Answer from the drawing. Dimensions are ordinates in mm from the lowest x, y and z of the part. Coordinates: 2 decimals unless noted, no trailing zeros. Write each loop counter-clockwise with the first axis right and the second up, starting at its lowest first coordinate (ties: lowest second). Pieces come first, ordered by that corner, then holes.
(1) Given pin 1 (5 mm diameter, centred on y = 18, z = 8.5, fed in from +X); pin 2 (4 mm diameter, centred on x = 69, z = 6, fed in from -Y); pin 3 (1.5 mm diameter, centred on y = 25, z = 3.5, fed in from +X) (1 decimal); pin 4 (4 mm diameter, centred on x = 96.5, z = 9.5, fed in from +Y), each flat-ended and moving along its own axis, determine where each tip first touches the part or whether it passes through.
(2) The part is cut by section D-D, the plane z = 2. Determine the outline of the cut face in (x, y) (1 decimal), and give its area (3 significant figures).
(3) Determine the mould class of the marked faces 1, 2, 3 and 4 for opening direction X: pulls with the +X half, pulls with the -X half, needs draft (parallel to the pull), parting line crosses it, or undercut.
(4) The part is cut by section A-A, the plane x = 12.7. Determine the outline of the cut face in (y, z).
(5) The part is cut by section C-C, the plane x = 114.3. Determine the outline of the cut face in (y, z).
(6) Straight lines are drawn through the part: line 1 along X through (y, z) = (31, 9.5); line 2 along Y through (x, z) = (122, 11.25); line 3 along Z through (x, y) = (87.5, 6.5) (1 decimal). For each, find the intervals that lie inside material, in ascending order.
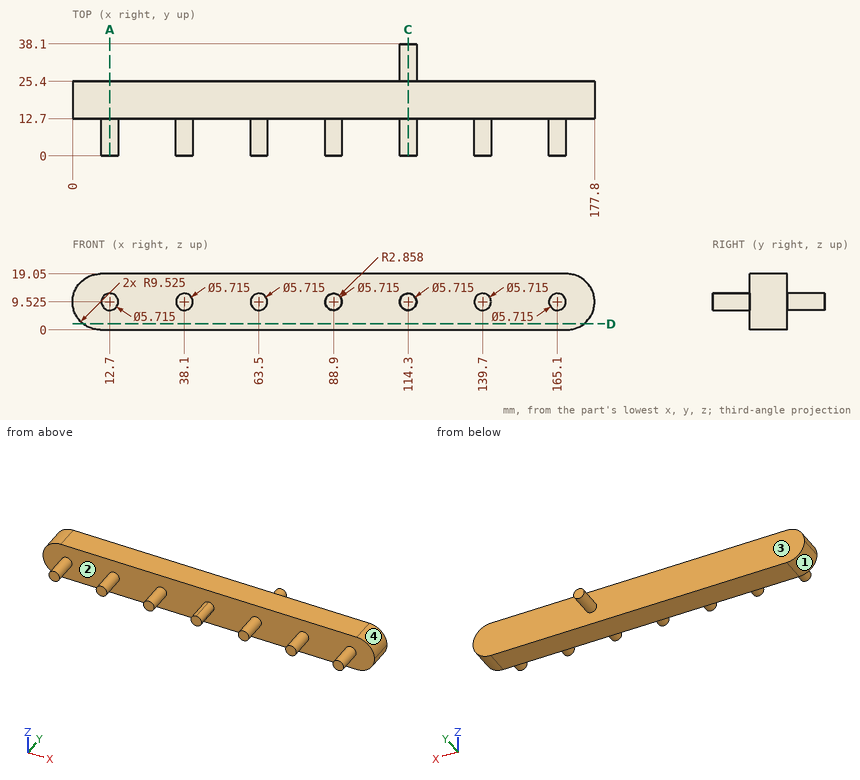
Computed:
1. pin 1: stops at x = 177.8
1. pin 2: stops at y = 12.7
1. pin 3: stops at x = 176.2
1. pin 4: stops at y = 25.4
2. outline: (3.7, 12.7) - (174.1, 12.7) - (174.1, 25.4) - (3.7, 25.4) - close
2. area: 2,160 mm2
3. face 1: pulls with the -X half
3. face 2: undercut
3. face 3: needs draft
3. face 4: pulls with the +X half
4. outline: (0, 6.67) - (12.7, 6.67) - (12.7, 0) - (25.4, 0) - (25.4, 19.05) - (12.7, 19.05) - (12.7, 12.38) - (0, 12.38) - close
5. outline: (0, 6.67) - (12.7, 6.67) - (12.7, 0) - (25.4, 0) - (25.4, 6.67) - (38.1, 6.67) - (38.1, 12.38) - (25.4, 12.38) - (25.4, 19.05) - (12.7, 19.05) - (12.7, 12.38) - (0, 12.38) - close
6. line 1: x = 111.44 to 117.16
6. line 2: y = 12.7 to 25.4
6. line 3: z = 7 to 12
